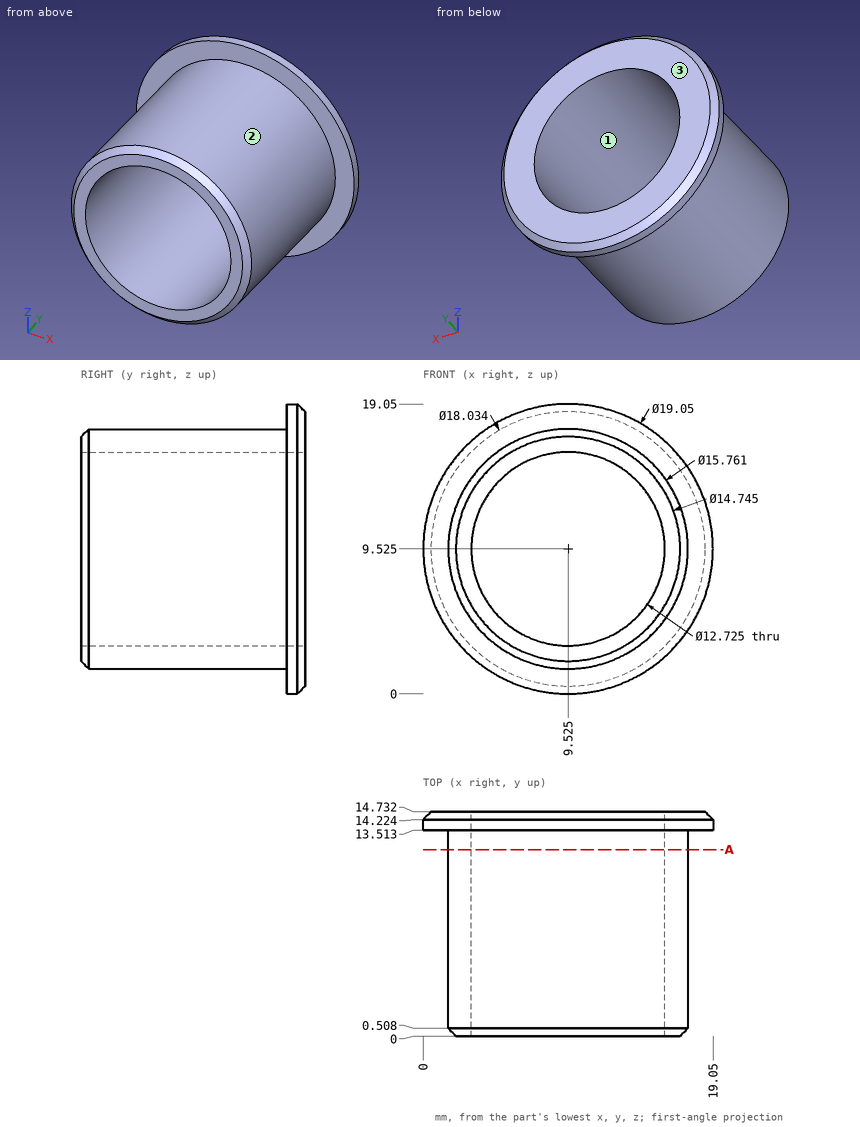
Answer from the drawing. Dimensions are ordinates in mm from the lowest x, y and z of the part. Give positions to 0.01 mm unless a question says otherwise; leave off trailing zeros. Order: outer loops, then holes, each group sorted by start corner. A loop starts at its lowest first (then second) coordinate and runs counter-clockwise, first axis right, second up. Notation, with made-up numbers: (-36.5, 38) -> (8.5, 38) arc R22 cw to (8.5, 44) -> close; hole circle Ø7 at (48.5, -22). An arc over 180 degrees is marked (long way). Answer as a JSON object with one key per item and string values. Group by question number.
1. Consider line 1 along X through (y, z) = (1.75, 9.25); line 2 along Z through (x, y) = (7, 3.75) (1 decimal); line 3 along X through (y, z) = (2.25, 12.5). Determine where each line is inside the solid, lowest interval first. Write a range as [from, to].
2. Section A-A on y = 12.25 is taken. Determine the outline of the cut face in (x, z) (1 decimal).
3. Flat-ended cylindrical pins translate along their axes: pin 1 Ø4 at (x, y) = (15.5, 3.5) entering from -Z; pin 2 Ø4 at (x, y) = (15, 7) entering from -Z; pin 3 Ø5 at (x, z) = (5.5, 5.5) entering from -Y; pin 4 Ø5 at (x, y) = (2.5, 12.5) entering from +Z. Find the tip coordinate at first contact, or state that the pin passes through.
4. The mould has two halves that part along Z. Classify the marked faces 1, 2 and 3: released by +Z, released by -Z, zero draft, split by the parting line, or undercut.
Result sheet:
{
 "1": {"line 1": "x = [1.65, 3.17], [15.88, 17.4]", "line 2": "z = [2.1, 3.7], [15.4, 17]", "line 3": "x = [2.23, 3.9], [15.15, 16.82]"},
 "2": {"outline": "circle Ø15.8 at (9.5, 9.5); hole circle Ø12.7 at (9.5, 9.5)"},
 "3": {"pin 1": "stops at z = 2.72", "pin 2": "stops at z = 2.45", "pin 3": "stops at y = 0", "pin 4": "stops at z = 17.79"},
 "4": {"face 1": "undercut", "face 2": "split by the parting line", "face 3": "zero draft"}
}
